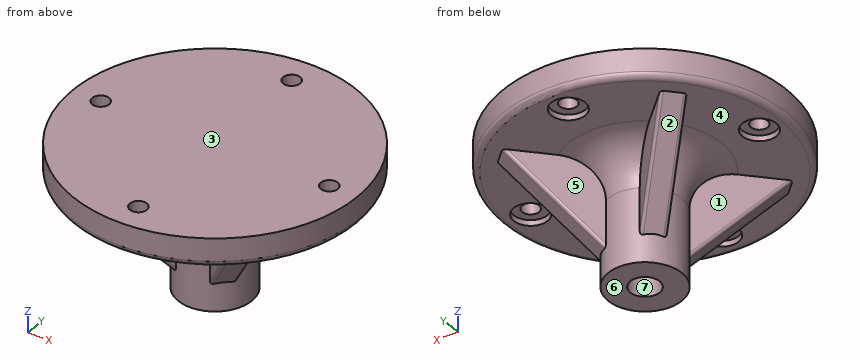
from build123d import *

# Parameters (mm, degrees)
SKETCH1_R           = 6.5
BOSS_EXTRUDE1_DEPTH = 20
SKETCH4_R           = 2.6
CUT_EXTRUDE1_DEPTH  = 15.5
FILLET1_R           = 1
SKETCH5_R           = 25
BOSS_EXTRUDE2_DEPTH = 5
CUT_EXTRUDE2_REACH  = 42.62
SKETCH6_R           = 1.5
FILLET2_R           = 7
RIB10_REACH         = 45.301
SKETCH12_WALL_W     = 109.815743814
SKETCH12_WALL_H     = 4
CIRPATTERN1_COUNT   = 4
FILLET3_R           = 1
FILLET4_R           = 0.5
SKETCH13_R          = 3
CUT_EXTRUDE3_DEPTH  = 1


with BuildPart() as part:
    # Sketch1 → Boss-Extrude1 (new body)
    with BuildSketch(Plane.XY):
        Circle(SKETCH1_R)
    extrude(amount=BOSS_EXTRUDE1_DEPTH)

    # Sketch4 → Cut-Extrude1 (cut)
    with BuildSketch(Plane(origin=(0, 0, 0), x_dir=(-1, 0, 0), z_dir=(0, 0, -1))):
        Circle(SKETCH4_R)
    extrude(amount=-CUT_EXTRUDE1_DEPTH, mode=Mode.SUBTRACT)

    # Fillet1
    fillet1_edges = [part.edges().sort_by_distance(p)[0] for p in [
        (2.6, 0, 15.5),
    ]]
    fillet(fillet1_edges, radius=FILLET1_R)

    # Sketch5 → Boss-Extrude2 (add)
    with BuildSketch(Plane.XY.offset(20)):
        Circle(SKETCH5_R)
    extrude(amount=BOSS_EXTRUDE2_DEPTH)

    # Sketch6 → Cut-Extrude2 (cut, up to next)
    with BuildSketch(Plane(origin=(0, 0, 20), x_dir=(-1, 0, 0), z_dir=(0, 0, -1)), mode=Mode.PRIVATE) as cut_extrude2_sk1:
        with Locations((0, 20)):
            Circle(SKETCH6_R)
    cut_extrude2_tool1 = extrude(cut_extrude2_sk1.sketch, amount=-CUT_EXTRUDE2_REACH, mode=Mode.PRIVATE) & part.part
    # Sketch6 → Cut-Extrude2 (cut, up to next)
    with BuildSketch(Plane(origin=(0, 0, 20), x_dir=(-1, 0, 0), z_dir=(0, 0, -1)), mode=Mode.PRIVATE) as cut_extrude2_sk2:
        with Locations((0, -20)):
            Circle(SKETCH6_R)
    cut_extrude2_tool2 = extrude(cut_extrude2_sk2.sketch, amount=-CUT_EXTRUDE2_REACH, mode=Mode.PRIVATE) & part.part
    # Sketch6 → Cut-Extrude2 (cut, up to next)
    with BuildSketch(Plane(origin=(0, 0, 20), x_dir=(-1, 0, 0), z_dir=(0, 0, -1)), mode=Mode.PRIVATE) as cut_extrude2_sk3:
        with Locations((-20, 0)):
            Circle(SKETCH6_R)
    cut_extrude2_tool3 = extrude(cut_extrude2_sk3.sketch, amount=-CUT_EXTRUDE2_REACH, mode=Mode.PRIVATE) & part.part
    # Sketch6 → Cut-Extrude2 (cut, up to next)
    with BuildSketch(Plane(origin=(0, 0, 20), x_dir=(-1, 0, 0), z_dir=(0, 0, -1)), mode=Mode.PRIVATE) as cut_extrude2_sk4:
        with Locations((20, 0)):
            Circle(SKETCH6_R)
    cut_extrude2_tool4 = extrude(cut_extrude2_sk4.sketch, amount=-CUT_EXTRUDE2_REACH, mode=Mode.PRIVATE) & part.part
    add(cut_extrude2_tool1.solids().sort_by_distance((0, 20, 20))[0], mode=Mode.SUBTRACT)
    add(cut_extrude2_tool2.solids().sort_by_distance((0, -20, 20))[0], mode=Mode.SUBTRACT)
    add(cut_extrude2_tool3.solids().sort_by_distance((20, 0, 20))[0], mode=Mode.SUBTRACT)
    add(cut_extrude2_tool4.solids().sort_by_distance((-20, 0, 20))[0], mode=Mode.SUBTRACT)

    # Fillet2
    fillet2_edges = [part.edges().sort_by_distance(p)[0] for p in [
        (-6.5, 0, 20),
    ]]
    fillet(fillet2_edges, radius=FILLET2_R)

    # Sketch12 wall → Rib10 (add, up to next)
    with BuildSketch(Plane(origin=(9.899494937, 9.899494937, 12.5), x_dir=(0.500000000005, 0.500000000005, 0.70710678118), z_dir=(0.499999999995, 0.499999999995, -0.707106781193)), mode=Mode.PRIVATE) as rib10_sk1:
        Rectangle(SKETCH12_WALL_W, SKETCH12_WALL_H)
    rib10_tool1 = extrude(rib10_sk1.sketch, amount=-RIB10_REACH, mode=Mode.PRIVATE) - part.part
    rib10 = rib10_tool1.solids().sort_by_distance((9.899494937, 9.899494937, 12.5))[0]
    add(rib10)

    # CirPattern1: Rib10 ×4 about axis
    cirpattern1_axis = Axis((0, 0, 0), (0, 0, 1))
    for i in range(1, CIRPATTERN1_COUNT):
        add(rib10.rotate(cirpattern1_axis, i * 360 / CIRPATTERN1_COUNT))

    # Fillet3
    fillet3_edges = [part.edges().sort_by_distance(p)[0] for p in [
        (-25, 0, 20),
    ]]
    fillet(fillet3_edges, radius=FILLET3_R)

    # Fillet4
    fillet4_edges = [part.edges().sort_by_distance(p)[0] for p in [
        (8.373791296, -11.202218421, 12.342329219),
        (11.202218421, -8.373791296, 12.342329219),
        (-8.373791296, -11.202218421, 12.342329219),
        (-11.202218421, -8.373791296, 12.342329219),
        (11.202218421, 8.373791296, 12.342329219),
        (8.373791296, 11.202218421, 12.342329219),
        (-11.202218421, 8.373791296, 12.342329219),
        (-8.373791296, 11.202218421, 12.342329219),
    ]]
    fillet(fillet4_edges, radius=FILLET4_R)

    # Sketch13 → Cut-Extrude3 (cut)
    with BuildSketch(Plane(origin=(0, 0, 20), x_dir=(-1, 0, 0), z_dir=(0, 0, -1))):
        with Locations((-20, 0)):
            Circle(SKETCH13_R)
        with Locations((0, 20)):
            Circle(SKETCH13_R)
        with Locations((20, 0)):
            Circle(SKETCH13_R)
        with Locations((0, -20)):
            Circle(SKETCH13_R)
    extrude(amount=-CUT_EXTRUDE3_DEPTH, mode=Mode.SUBTRACT)


solid = part.part
CAD build for the part. Positions are in the model's coordinates, mm. Face numbers are marked on the shaded views. A direction names the side the tool comes from. Give positions to 0.01 mm unless a question says otherwise; leave off trailing zeros. Write each loop counter-clockwise with the first axis right and the second up, starting at its lowest first coordinate (ties: lowest second). Pieces come first, ordered by that corner, then holes. Notation, with made-up numbers: (12.5, 60.5) - (22.5, 60.5) arc R23 cw to (22.5, 82.5) - close; hole circle Ø11 at (27.25, 68.5). An arc over 180 degrees is marked (long way). Put each result on its own line as item: value.
(1) Wall check: L1, parallel to Y at x = 0, z = 9.75; L2, parallel to Y at x = 20, z = 23.2; L3, parallel to Y at x = 0, z = 20.7. Give the ranges that are in metal, low to high.
Working result:
L1: -6.5 to -2.6, 2.6 to 6.5
L2: -15 to -1.5, 1.5 to 15
L3: -24.95 to -23, -17 to 17, 23 to 24.95
(2) Saw through at A-A (y = 0). Count the separate pieces of the cut face and the enclosed holes in it, then the cut area to 3 significant figures.
Working result:
separate pieces: 3
enclosed holes: 0
area: 414 mm^2
(3) Drop flat-ended pins along their axis: pin 1 Ø6.5 at (x, y) = (-20, 1) entering from -Z; pin 2 Ø5 at (x, y) = (0, 20) entering from -Z; pin 3 Ø3 at (y, z) = (6.5, 19) entering from +X. Give the stop position or say it passes through.
Working result:
pin 1: z = 20
pin 2: z = 21
pin 3: x = 24.07
(4) Tool access for the marked faces 5, 6 and 7: list every direction of +Z, -Z, +X, -X, +Y, -Y with a clear straight run to the whole face (end or side of a thin tool).
Working result:
face 5: -Z, +Y
face 6: -Z, +X, -X, +Y, -Y
face 7: -Z
(5) Saw through at B-B (z = 2.75). List the corners of the cut face in (x, y).
Working result:
outline: circle Ø13 at (0, 0); hole circle Ø5.2 at (0, 0)
(6) Pull direction Y, two halves, no side cores. Call the marked faces 1, 2, 3 and 4: released by +Y, released by -Y, zero draft, split by the parting line, or undercut.
Working result:
face 1: undercut
face 2: released by +Y
face 3: zero draft
face 4: undercut
